Check sheet for the modelled part. Datum: model origin and axes. Units: mm. A direction names the side the tool comes from. Coordinates: 2 decimals unless noted, no trailing zeros. Loops run counter-clockwise (first coordinate to the right, second up) from the corner with the lowest first, then second, coordinate; pieces in that order, holes last. Notation, with made-up numbers: (16, 29.5) -> (36, 29.5) arc R12 cw to (36, 41.5) -> close; hole circle Ø9 at (49, 2.5). An arc over 180 degrees is marked (long way). Use one line per item in the form item = value.
from build123d import *
from build123d.topology import SkipClean

# Parameters (mm, degrees)
SKETCH1_R           = 0.75
BOSS_EXTRUDE1_DEPTH = 2.08
SKETCH2_R           = 3.375
BOSS_EXTRUDE2_DEPTH = 2.31
SKETCH3_R           = 2.25
CUT_EXTRUDE1_DEPTH  = 0.84


with BuildPart() as part:
    # Sketch1 → Boss-Extrude1 (new body)
    with BuildSketch(Plane(origin=(0, 0, 0), x_dir=(1, 0, 0), z_dir=(0, 1, 0))):
        with BuildLine():
            Line((0.28743419, 3.36273796), (16.315331372, 1.992733606))
            ThreePointArc((16.315331372, 1.992733606), (18.145, 0), (16.315331372, -1.992733606))
            Line((16.315331372, -1.992733606), (0.28743419, -3.36273796))
            ThreePointArc((0.28743419, -3.36273796), (-3.375, 0), (0.28743419, 3.36273796))
        make_face()
        with Locations(Location((16.605, 0, 0), (0, 0, 270))):
            Circle(SKETCH1_R, mode=Mode.SUBTRACT)
    extrude(amount=BOSS_EXTRUDE1_DEPTH)

    # Sketch2 → Boss-Extrude2 (add)
    with SkipClean():  # the faces are left unmerged after this step: merging them gives an invalid solid
        with BuildSketch(Plane(origin=(0, 2.08, 0), x_dir=(1, 0, 0), z_dir=(0, 1, 0))):
            with Locations(Location((0, 0, 0), (0, 0, 85.114447475))):
                Circle(SKETCH2_R)
        extrude(amount=BOSS_EXTRUDE2_DEPTH)

    # Sketch3 → Cut-Extrude1 (cut)
    with SkipClean():  # the faces are left unmerged after this step: merging them gives an invalid solid
        with BuildSketch(Plane(origin=(0, 0, 0), x_dir=(1, 0, 0), z_dir=(0, 1, 0))):
            with Locations(Location((0, 0, 0), (0, 0, 270))):
                Circle(SKETCH3_R)
        extrude(amount=CUT_EXTRUDE1_DEPTH, mode=Mode.SUBTRACT)


solid = part.part
(1) Section check D-D, the plane z = -1. Record the boundary of the cut face in (x, y).
Established:
outline = (-3.22, 0) -> (-2.02, 0) -> (-2.02, 0.84) -> (2.02, 0.84) -> (2.02, 0) -> (17.88, 0) -> (17.88, 2.08) -> (3.22, 2.08) -> (3.22, 4.39) -> (-3.22, 4.39) -> close
(2) Tool access check on faces 4 (the cylindrical face through (0.676, 0.414, 2.146)), 5 (the flat face through (8.41, 1.03, 2.67)). Record the directions out of +Z, -Z, +X, -X, +Y, -Y that give a thin tool (end or side, any length) a straight path to the whole face; none if there is none.
Established:
face_4 = -Y
face_5 = +Z, +X, +Y, -Y
(3) Scan lines: line 1 along X through (y, z) = (0.8, 0) (3 decimals); line 2 along X through (y, z) = (1, 0) (3 decimals); line 3 along Y through (x, z) = (7.5, 1.5). Record each from-to range of solid material in increasing order.
Established:
line_1 = -3.375 to -2.25, 2.25 to 15.855, 17.355 to 18.145
line_2 = -3.375 to 15.855, 17.355 to 18.145
line_3 = 0 to 2.08
(4) Section check B-B, the plane x = 0. Record the boundary of the cut face in (y, z) (3 decimals), plus the area to 3 significant figures.
Established:
outline = (0, -3.375) -> (4.39, -3.375) -> (4.39, 3.375) -> (0, 3.375) -> (0, 2.25) -> (0.84, 2.25) -> (0.84, -2.25) -> (0, -2.25) -> close
area = 25.9 mm²
(5) Section check A-A, the plane z = 0. Record the boundary of the cut face in (x, y) (3 decimals).
Established:
outline = (-3.375, 0) -> (-2.25, 0) -> (-2.25, 0.84) -> (2.25, 0.84) -> (2.25, 0) -> (15.855, 0) -> (15.855, 2.08) -> (3.375, 2.08) -> (3.375, 4.39) -> (-3.375, 4.39) -> close; (17.355, 0) -> (18.145, 0) -> (18.145, 2.08) -> (17.355, 2.08) -> close
(6) Go/stop test with a flat-tipped pin: P1, Ø2, axis at x = 16.605, z = 0, coming from the +Y side. Record where the tip stops, or that it passes through.
Established:
P1 = 2.08
(7) Mould release check, pull along Z, two halves, no side actions. Record for faces 1 (the cylindrical face through (18.145, 1.025, -0.042)), 2 (the flat face through (8.189, 1.025, -2.687)), 3 (the flat face through (0, 0.84, 0)): +Z half, -Z half, draft (parallel to the pull), parting line (faces both ways), or undercut.
Established:
face_1 = parting line
face_2 = -Z half
face_3 = undercut
(8) Section check C-C, the plane y = 3.6. Record the boundary of the cut face in (x, z) (3 decimals).
Established:
outline = circle Ø6.75 at (0, 0)
